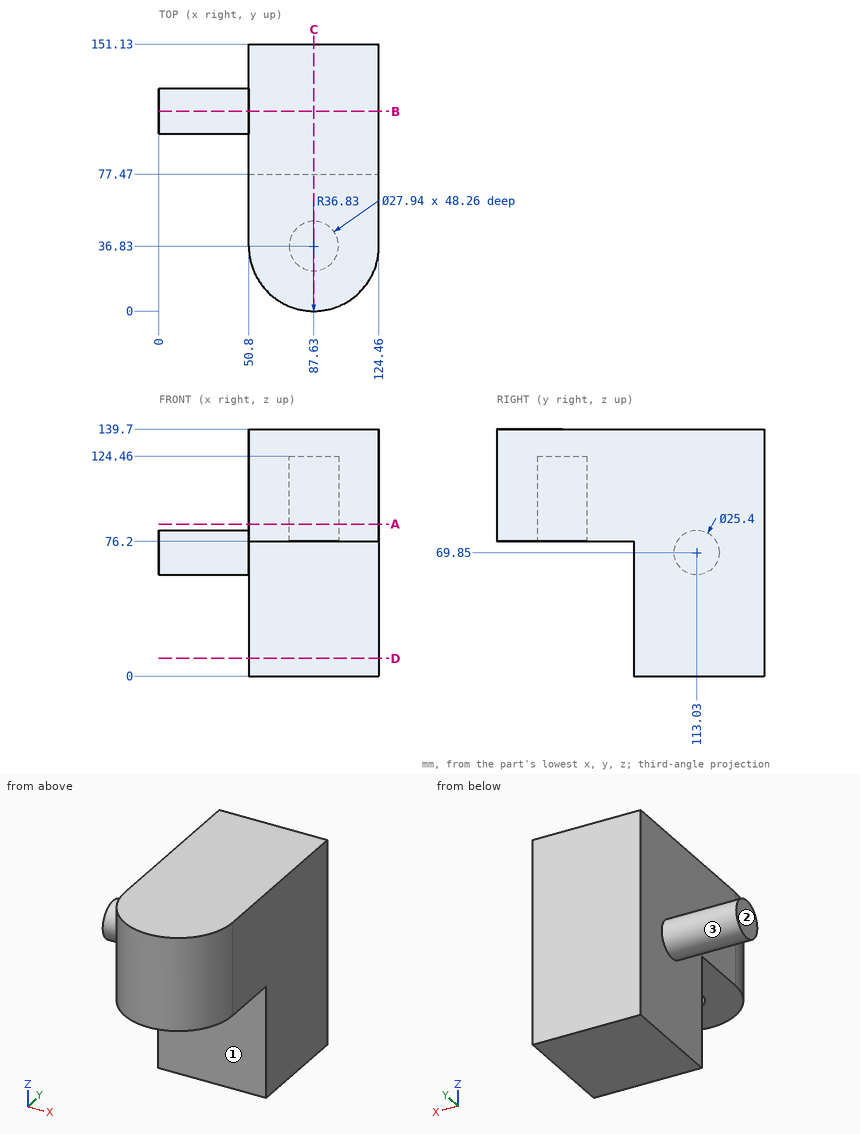
The figure shows three views and two pictorial views of one solid part (mm, origin at its lowest corner). Answer the questions. A direction names the side the tool comes from. Round coordinates to 2 decimals unless told otherwise and drop trailing zeros. Write each loop counter-clockwise with the first axis right and the second up, starting at its lowest first coordinate (ties: lowest second). Pieces come first, ordered by that corner, then holes. Notation, with made-up numbers: (48, 15.5) - (85, 15.5) arc R26 ccw to (85, 42.5) - close; hole circle Ø10 at (64.25, 44). An arc over 180 degrees is marked (long way). One line per question, with ' | ' between items. Start each with the question number.
1. Each of these flat-tipped pins is pushed along its axis until it touches: pin 1 (25 mm diameter, centred on x = 87.63, y = 36.83, fed in from -Z); pin 2 (12 mm diameter, centred on x = 93, z = 77.5, fed in from -Y); pin 3 (12 mm diameter, centred on x = 95, z = 69, fed in from -Y); pin 4 (6 mm diameter, centred on x = 79, y = 130.5, fed in from -Z). Where does it stop, or does it pass through?
2. Section D-D (z = 10) is taken. Determine the outline of the cut face in (x, y), and give its area (3 significant figures).
3. Section A-A (z = 86) is taken. Determine the outline of the cut face in (x, y).
4. For the marked faces 1, 2 and 3, determine the directions among +Z, -Z, +X, -X, +Y, -Y from which every point of the face is accessible in a straight line to the end or side of a thin tool.
5. Find the intervals of material crossed by probe 1 along Y at (x, z) = (87.5, 99); probe 2 along X at (y, z) = (36, 106); probe 3 along X at (y, z) = (137.5, 126), in increasing order. Write a range as [from, to].
6. Section B-B (y = 113.03) is taken. Determine the outline of the cut face in (x, z), and give its area (3 significant figures).
7. Section C-C (x = 87.63) is taken. Determine the outline of the cut face in (y, z), and give its area (3 significant figures).
Filled in:
1) pin 1: z = 124.46 | pin 2: y = 0 | pin 3: y = 77.47 | pin 4: z = 0
2) outline: (50.8, 77.47) - (124.46, 77.47) - (124.46, 151.13) - (50.8, 151.13) - close | area: 5,430 mm²
3) outline: (50.8, 36.83) arc R36.83 ccw to (124.46, 36.83) - (124.46, 151.13) - (50.8, 151.13) - close; hole circle Ø27.94 at (87.63, 36.83)
4) face 1: -Z, +X, -X, -Y | face 2: +Z, -Z, -X, +Y, -Y | face 3: -X
5) probe 1: [0, 22.86], [50.8, 151.13] | probe 2: [50.81, 73.68], [101.58, 124.45] | probe 3: [50.8, 124.46]
6) outline: (0, 57.15) - (50.8, 57.15) - (50.8, 0) - (124.46, 0) - (124.46, 139.7) - (50.8, 139.7) - (50.8, 82.55) - (0, 82.55) - close | area: 11,600 mm²
7) outline: (0, 76.2) - (22.86, 76.2) - (22.86, 124.46) - (50.8, 124.46) - (50.8, 76.2) - (77.47, 76.2) - (77.47, 0) - (151.13, 0) - (151.13, 139.7) - (0, 139.7) - close | area: 13,900 mm²
